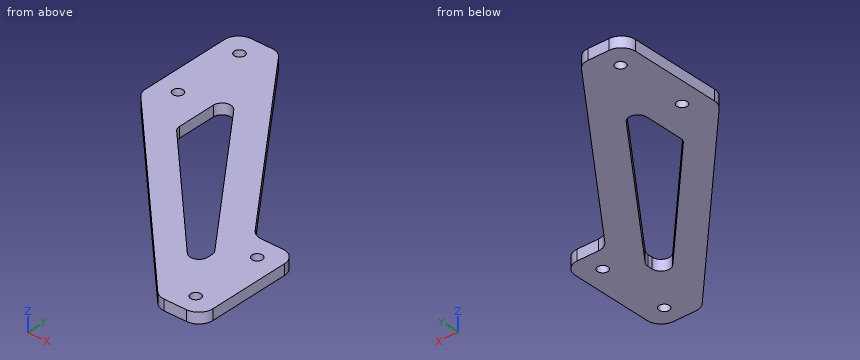
```python
from build123d import *

# Parameters (mm, degrees)
SKETCH_1_R          = 1.45
EXTRUDE_1_DEPTH     = 3
CUT_EXTRUDE_1_DEPTH = 3
FILLET_1_R          = 4
FILLET_2_R          = 2.5


with BuildPart() as part:
    # 草图1 → 凸台-拉伸1 (new body)
    with BuildSketch(Plane.XY):
        Polygon((-49, 63.5), (-61, 63.5), (-61, 32.199032391), (-6, -25.300967609), (6, -25.300967609), (6, 6), (-6, 6), align=None)
        Circle(SKETCH_1_R, mode=Mode.SUBTRACT)
        with Locations((0, -20)):
            Circle(SKETCH_1_R, mode=Mode.SUBTRACT)
        with Locations((-55, 37.5)):
            Circle(SKETCH_1_R, mode=Mode.SUBTRACT)
        with Locations((-55, 57.5)):
            Circle(SKETCH_1_R, mode=Mode.SUBTRACT)
    extrude(amount=EXTRUDE_1_DEPTH)

    # 草图2 → 切除-拉伸1 (cut)
    with BuildSketch(Plane.XY.offset(3)):
        Polygon((-46, 46.130219602), (-46, 26.644197231), (-8, -13.083075497), (-8, -4.683733886), align=None)
    extrude(amount=-CUT_EXTRUDE_1_DEPTH, mode=Mode.SUBTRACT)

    # 圆角1
    fillet_1_edges = [part.edges().sort_by_distance(p)[0] for p in [
        (-6, 6, 1.5),
        (6, 6, 1.5),
        (6, -25.300967609, 1.5),
        (-6, -25.300967609, 1.5),
        (-61, 32.199032391, 1.5),
        (-61, 63.5, 1.5),
        (-49, 63.5, 1.5),
    ]]
    fillet(fillet_1_edges, radius=FILLET_1_R)

    # 圆角2
    fillet_2_edges = [part.edges().sort_by_distance(p)[0] for p in [
        (-46, 46.130219602, 1.5),
        (-8, -4.683733886, 1.5),
        (-8, -13.083075497, 1.5),
        (-46, 26.644197231, 1.5),
    ]]
    fillet(fillet_2_edges, radius=FILLET_2_R)


solid = part.part
```
Geometry: final body of the model. Coordinates: model frame, mm. Give positions to 0.01 mm unless a question says otherwise; leave off trailing zeros. Order: outer loops, then holes, each group sorted by start corner. A loop starts at its lowest first (then second) coordinate and runs counter-clockwise, first axis right, second up. Notation, with made-up numbers: (30.5, 63.5) -> (51.5, 63.5) arc R13 cw to (51.5, 72.5) -> close; hole circle Ø11 at (-38, 37). An arc over 180 degrees is marked (long way). Write each question's results on one line, items separated by ' | '. Start each with the question number.
1) Section D-D (y = 37.5). Return loops of the section in (x, z), then the cut area to 3 significant figures.
2) Section C-C (x = 0). Return loops of the section in (y, z).
3) Section A-A (z = 0.6). Return loops of the section in (x, y), then the cut area to 3 significant figures.
4) First-contact query: pin 1 (0.7 mm diameter, centred on y = -6, z = 2, fed in from -X); pin 2 (12 mm diameter, centred on x = -34, y = 51.5, fed in from +Z); pin 3 (0.9 mm diameter, centred on y = 31, z = 1, fed in from +X). Flat tips, straight axial feed; report the tip coordinate or a pass-through.
5) Line query: line 1 (Y direction, x = -55, z = 1.8); line 2 (Y direction, x = 0, z = 1.5); line 3 (X direction, y = -1.5, z = 2.8). Output: solid intervals per line, ascending. Write a range as from..to.
6) Section B-B (y = -20). Return loops of the section in (x, z).
Calculated:
1) outline: (-61, 0) -> (-56.45, 0) -> (-56.45, 3) -> (-61, 3) -> close; (-53.55, 0) -> (-46, 0) -> (-46, 3) -> (-53.55, 3) -> close; (-39.55, 0) -> (-29.56, 0) -> (-29.56, 3) -> (-39.55, 3) -> close | area: 66.3 mm2
2) outline: (-25.3, 0) -> (-21.45, 0) -> (-21.45, 3) -> (-25.3, 3) -> close; (-18.55, 0) -> (-1.45, 0) -> (-1.45, 3) -> (-18.55, 3) -> close; (1.45, 0) -> (6, 0) -> (6, 3) -> (1.45, 3) -> close
3) outline: (-61, 33.8) arc R4 ccw to (-59.89, 31.04) -> (-7.18, -24.07) arc R4 ccw to (-4.29, -25.3) -> (2, -25.3) arc R4 ccw to (6, -21.3) -> (6, 2) arc R4 ccw to (2, 6) -> (-4, 6) arc R4 cw to (-7.2, 7.6) -> (-47.8, 61.9) arc R4 ccw to (-51, 63.5) -> (-57, 63.5) arc R4 ccw to (-61, 59.5) -> close; hole circle Ø2.9 at (-55, 37.5); hole circle Ø2.9 at (-55, 57.5); hole (-46, 27.65) arc R2.5 ccw to (-45.31, 25.92) -> (-12.31, -8.58) arc R2.5 ccw to (-8, -6.85) -> (-8, -5.52) arc R2.5 ccw to (-8.5, -4.02) -> (-41.5, 40.11) arc R2.5 ccw to (-46, 38.61) -> close; hole circle Ø2.9 at (0, -20); hole circle Ø2.9 at (0, 0) | area: 1,890 mm2
4) pin 1: x = -24.8 | pin 2: z = 3 | pin 3: x = -24.36
5) line 1: 25.93..36.05, 38.95..56.05, 58.95..63.5 | line 2: -25.3..-21.45, -18.55..-1.45, 1.45..6 | line 3: -28.77..-19.08, -10.38..6
6) outline: (-11.07, 0) -> (-1.45, 0) -> (-1.45, 3) -> (-11.07, 3) -> close; (1.45, 0) -> (6, 0) -> (6, 3) -> (1.45, 3) -> close
